Read the model definition and answer for the solid it produces. Units are mm, in the model's axes. A direction names the side the tool comes from. Round coordinates to 2 decimals unless told otherwise and drop trailing zeros. Order: outer loops, then holes, each group sorted by start corner. A loop starts at its lowest first (then second) coordinate and runs counter-clockwise, first axis right, second up. Notation, with made-up numbers: (72, -10) -> (91, -10) arc R19 ccw to (91, 8) -> close; hole circle Ø7 at (87, -36). An arc over 180 degrees is marked (long way). Use a Markdown table: item, result. Add a question column.
1. Consider L1, parallel to X at y = 12.5, z = -141; L2, parallel to X at y = 79.5, z = -560; L3, parallel to Z at x = 266, y = 86. Determine where each line is inside the solid, lowest interval first. Write a range as [from, to].
2. For faces 1 (the face through (309.724, 91.835, -710.478)), 2 (the face through (24, 49, 0)), determine the directions among +Z, -Z, +X, -X, +Y, -Y from which every point of the face is accessible in a straight line to the end or side of a thin tool.
3. Section A-A, the plane y = 99.5 is taken. Give the vertices of the cut face in (x, z), then the cut area to 3 significant figures.
4. Given pin 1 (5 mm diameter, centred on y = 120, z = -875.5, fed in from +X); pin 2 (10 mm diameter, centred on x = 757.5, y = 22.5, fed in from -Z) (3 decimals); pin 3 (5 mm diameter, centred on y = 86.5, z = -280.5, fed in from +X), each flat-ended and moving along its own axis, determine where each tip first touches the part or whether it passes through.
```python
from build123d import *

# Parameters (mm, degrees)
BOTTOM_LEVEL_DEPTH = 5
MID_LEVEL_DEPTH    = 35
GUARD_RAIL_DEPTH   = 100
ROUNDING_R         = 5


with BuildPart() as part:
    # Sketch1 → Bottom level (new body)
    with BuildSketch(Plane(origin=(0, 0, 0), x_dir=(1, 0, 0), z_dir=(0, 1, 0))):
        with BuildLine():
            Line((0, 0), (25, 0))
            ThreePointArc((25, 0), (321.11504422, 714.88495578), (1036, 1011))
            Line((1036, 1011), (1036, 1036))
            ThreePointArc((1036, 1036), (303.437374691, 732.562625309), (0, 0))
        make_face()
    extrude(amount=BOTTOM_LEVEL_DEPTH)

    # Sketch2 → Mid level (add)
    with BuildSketch(Plane(origin=(0, 5, 0), x_dir=(1, 0, 0), z_dir=(0, 1, 0))):
        with BuildLine():
            Line((1036, 1011), (1036, 1026))
            ThreePointArc((1036, 1026), (310.508442503, 725.491557497), (10, 0))
            Line((10, 0), (25, 0))
            ThreePointArc((25, 0), (321.11504422, 714.88495578), (1036, 1011))
        make_face()
    extrude(amount=MID_LEVEL_DEPTH)

    # Sketch3 → Guard rail (add)
    with BuildSketch(Plane(origin=(0, 40, 0), x_dir=(1, 0, 0), z_dir=(0, 1, 0))):
        with BuildLine():
            Line((1036, 1016), (1036, 1011))
            ThreePointArc((1036, 1011), (321.11504422, 714.88495578), (25, 0))
            Line((25, 0), (20, 0))
            ThreePointArc((20, 0), (317.579510314, 718.420489686), (1036, 1016))
        make_face()
    extrude(amount=GUARD_RAIL_DEPTH)

    # Rounding
    rounding_edges = [part.edges().sort_by_distance(p)[0] for p in [
        (317.579510314, 40, -718.420489686),
        (310.508442503, 40, -725.491557497),
        (310.508442503, 5, -725.491557497),
    ]]
    fillet(rounding_edges, radius=ROUNDING_R - 0.0001)  # a hair under: the kernel refuses the full size


solid = part.part
```
Verdict:
| question | item | result |
|---|---|---|
| 1 | L1 | x = [19.73, 34.88] |
| 1 | L2 | x = [188.26, 194.26] |
| 1 | L3 | z = [-662.84, -655.15] |
| 2 | face 1 | -Z, -X, +Y |
| 2 | face 2 | +Z, +X, -X, +Y, -Y |
| 3 | outline | (20, 0) arc R1016 ccw to (1036, -1016) -> (1036, -1011) arc R1011 cw to (25, 0) -> close |
| 3 | area | 7,960 mm2 |
| 4 | pin 1 | stops at x = 534.76 |
| 4 | pin 2 | stops at z = -988.875 |
| 4 | pin 3 | stops at x = 65.42 |
